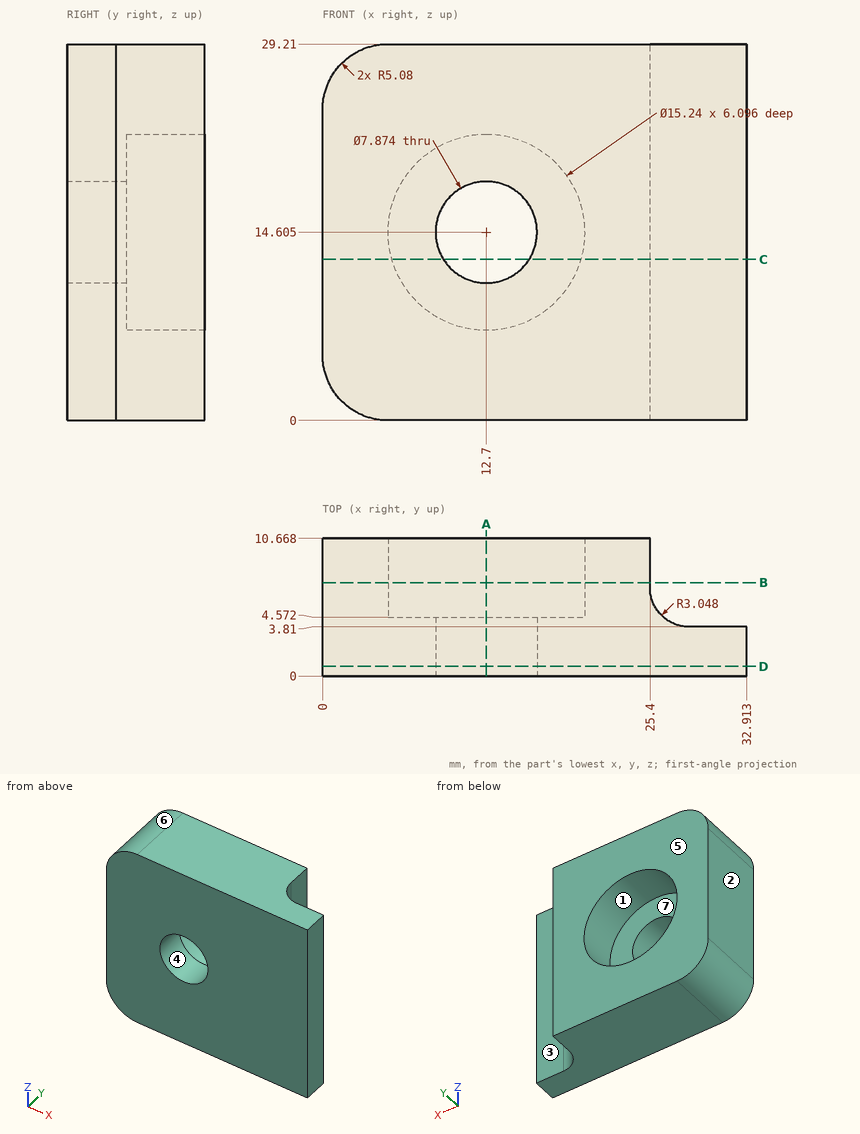
Print and shaded views of the part. All mm, measured from the part's lowest x, y and z. A direction names the side the tool comes from. Round coordinates to 2 decimals unless told otherwise and drop trailing zeros. Order: outer loops, then holes, each group sorted by start corner. A loop starts at its lowest first (then second) coordinate and runs counter-clockwise, first axis right, second up.
Q1. Slice it at B-B (y = 7.25). Write the cut outline in (x, z) (3 decimals).
Q2. Drop flat-ended pins along their axis: pin 1 (6 mm diameter, centred on y = 5.5, z = 6.5, fed in from -X); pin 2 (5 mm diameter, centred on x = 31.5, z = 13, fed in from +Y); pin 3 (4 mm diameter, centred on y = 8.5, z = 9.5, fed in from +X). Give the stop position or say it passes through.
Q3. Wall check: L1, parallel to Z at x = 12.7, y = 6.25 (3 decimals); L2, parallel to Y at x = 29.5, z = 12; L3, parallel to Z at x = 12, y = 0.5. Give the ranges that are in metal, low to high.
Q4. Two-plate mould, pull along Z, no slides. Class the marked faces 4, 5, 6 and 7: pulls with the +Z half, pulls with the -Z half, needs draft (parallel to the pull), parting line crosses it, or undercut.
Q5. Which spindle directions (+Z, -Z, +X, -X, +Y, -Y) get a long thin tool onto all of the face, cutting with end or side? Do the marked faces 1, 2 and 3. Say none if no direction does.
Q6. Slice it at A-A (x = 12.7). Write the cut outline in (y, z) (3 decimals), and give its area (3 significant figures).
Q7. Slice it at D-D (y = 0.75). Write the cut outline in (x, z) (3 decimals).
Q8. Slice it at C-C (z = 12.5). Write the cut outline in (x, y).
Results below:
1. outline: (0, 5.08) arc R5.08 ccw to (5.08, 0) - (25.4, 0) - (25.4, 29.21) - (5.08, 29.21) arc R5.08 ccw to (0, 24.13) - close; hole circle Ø15.24 at (12.7, 14.605)
2. pin 1: stops at x = 0
2. pin 2: stops at y = 3.81
2. pin 3: stops at x = 25.42
3. L1: z = 0 to 6.985, 22.225 to 29.21
3. L2: y = 0 to 3.81
3. L3: z = 0 to 10.73, 18.48 to 29.21
4. face 4: undercut
4. face 5: needs draft
4. face 6: pulls with the +Z half
4. face 7: undercut
5. face 1: +Y
5. face 2: +Z, -Z, -X, +Y, -Y
5. face 3: +Z, -Z, +X, +Y
6. outline: (0, 0) - (10.668, 0) - (10.668, 6.985) - (4.572, 6.985) - (4.572, 10.668) - (0, 10.668) - close; (0, 18.542) - (4.572, 18.542) - (4.572, 22.225) - (10.668, 22.225) - (10.668, 29.21) - (0, 29.21) - close
6. area: 183 mm2
7. outline: (0, 5.08) arc R5.08 ccw to (5.08, 0) - (32.913, 0) - (32.913, 29.21) - (5.08, 29.21) arc R5.08 ccw to (0, 24.13) - close; hole circle Ø7.874 at (12.7, 14.605)
8. outline: (0, 0) - (9.37, 0) - (9.37, 4.57) - (5.38, 4.57) - (5.38, 10.67) - (0, 10.67) - close; (16.03, 0) - (32.91, 0) - (32.91, 3.81) - (28.45, 3.81) arc R3.05 cw to (25.4, 6.86) - (25.4, 10.67) - (20.02, 10.67) - (20.02, 4.57) - (16.03, 4.57) - close
